from build123d import *

# Parameters (mm, degrees)
F0_W      = 184.15
F0_H      = 50.8
F1_DEPTH  = 8.128
F3_D      = 5.1054
F6_D      = 4.9784
F7_W      = 76.2
F7_H      = 9.525
F8_DEPTH  = 8.129
F9_SIZE   = 9.525
F10_SIZE  = 2.54
F15_DEPTH = 25.4
F17_D     = 5.1054
F18_R     = 2.4892
F19_DEPTH = 4.064
F20_SIZE  = 4.06399


# Not quite as in the source:
# - a fillet or chamfer is up to 0.001 mm smaller than in the source, because OpenCascade refuses the exact size
# - a feature names something its author has since deleted; it is built from what else it names


with BuildPart() as f1:
    # F0 (on Top) → F1 (new body)
    with BuildSketch(Plane.XY):
        Rectangle(F0_W, F0_H)
    extrude(amount=F1_DEPTH)

    # F3 (through all)
    with Locations(Plane.XY.offset(8.128)):
        with Locations((-60.325, 12.7), (-76.2, -12.7), (-44.45, -12.7)):
            Hole(F3_D / 2)

    # F6 (through all)
    with Locations(Plane.XY.offset(8.128)):
        with Locations((79.375, 12.7), (79.375, -12.7)):
            Hole(F6_D / 2)

    # F7 (on face) → F8 (cut, through all)
    with BuildSketch(Plane.XY.offset(8.128)):
        Polygon((66.675, 25.4), (-47.625, 25.4), (-34.925, 12.7), (53.975, 12.7), align=None)
        with Locations((15.875, -4.7625)):
            Rectangle(F7_W, F7_H)
    extrude(amount=-F8_DEPTH, mode=Mode.SUBTRACT)

    # F9
    f9_edges = [f1.edges().sort_by_distance(p)[0] for p in [
        (-92.075, -25.4, 4.064),
        (-92.075, 25.4, 4.064),
        (92.075, -25.4, 4.064),
        (92.075, 25.4, 4.064),
    ]]
    chamfer(f9_edges, length=F9_SIZE)

    # F10
    f10_edges = [f1.edges().sort_by_distance(p)[0] for p in [
        (-22.225, 0, 4.064),
        (-22.225, -9.525, 4.064),
        (53.975, 0, 4.064),
        (53.975, -9.525, 4.064),
    ]]
    chamfer(f10_edges, length=F10_SIZE)


with BuildPart() as f13_1:
    # F13: instance of F1
    add(f1.part.mirror(Plane(origin=(92.075, 0, 4.064), x_dir=(0, 1, 0), z_dir=(1, 0, 0))))

    # F17 (through all)
    with Locations(Plane.XY.offset(8.128)):
        with Locations((244.475, -6.35)):
            Hole(F17_D / 2)

    # F18 (on face) → F19 (cut)
    with BuildSketch(Plane(origin=(0, 0, 0), x_dir=(1, 0, 0), z_dir=(0, 0, -1))):
        Polygon((125.095, 25.4), (117.475, 25.4), (101.6, 25.4), (92.075, 15.875), (92.075, -15.875), (101.6, -25.4), (117.475, -25.4), (125.095, -17.78), align=None)
        with Locations((104.775, -12.7)):
            Circle(F18_R, mode=Mode.SUBTRACT)
        with Locations((104.775, 12.7)):
            Circle(F18_R, mode=Mode.SUBTRACT)
    extrude(amount=-F19_DEPTH, mode=Mode.SUBTRACT)

    # F20 (size 4.064 in the source; OpenCascade refuses exactly that, so slightly less here)
    f20_edges = [f13_1.edges().sort_by_distance(p)[0] for p in [
        (125.095, -3.81, 4.064),
    ]]
    chamfer(f20_edges, length=F20_SIZE)


with BuildPart() as f1_1:
    add(f1.part)

    # F14 (on face) → F15 (cut)
    with BuildSketch(Plane.XY.offset(8.128)):
        Polygon((-100.5587801337, -25.4), (92.075, -25.4), (92.075, -15.875), (92.075, 15.875), (92.075, 34.0131297708), (-100.5587801337, 34.0131297708), align=None)
    extrude(amount=-F15_DEPTH, mode=Mode.SUBTRACT)


solid = f13_1.part
Input: part model. Units: mm. Frame: model coordinates. A direction names the side the tool comes from. Give positions to 0.01 mm unless a question says otherwise; leave off trailing zeros. Loops run counter-clockwise (first coordinate to the right, second up) from the corner with the lowest first, then second, coordinate; pieces in that order, holes last. Notation, with made-up numbers: M -9.75,-32 L 5.25,-32 A12 ccw 5.25,-22 Z; hole C 30.25,66 d9. An arc over 180 degrees is marked long. Use CSV: the item, a comma, the result in double quotes.
(1) Section A-A, the plane y = -12.7. Count the separate pieces of the cut face and the enclosed holes in it, plus the area to 3 significant figures.
Outcome:
separate pieces,"4"
enclosed holes,"0"
area,"1,270 mm²"
(2) Section C-C, the plane x = 260.35. Return loops of the section in (y, z).
Outcome:
outline,"M -25.4,0 L -15.25,0 L -15.25,8.13 L -25.4,8.13 Z; M -10.15,0 L 25.4,0 L 25.4,8.13 L -10.15,8.13 Z"
(3) Pull-direction query (X, two-part tool) for faces 4 (the face through (130.175, -5, 4)), 5 (the face through (169, -9.525, 4)), 6 (the face through (185.4, 0.4, 8.128)), 7 (the face through (123.035, -1.447, 2.06)); classes: pulls with the +X half, pulls with the -X half, needs draft (parallel to the pull), parting line crosses it, or undercut.
Outcome:
face 4,"undercut"
face 5,"undercut"
face 6,"needs draft"
face 7,"pulls with the -X half"
(4) Set-up query: faces 1 (the face through (169, 0, 4)), 2 (the face through (125.325, 17.55, 5.024)), 3 (the face through (185, -25.4, 4)). Return all of +Z, -Z, +X, -X, +Y, -Y with unobstructed straight access to the full face (end or side cutting, diameter ignored); none if empty.
Outcome:
face 1,"+Z, -Z"
face 2,"+Z, -Z, +Y"
face 3,"+Z, -Z, +X, -X, -Y"
(5) Pin query (flat end, axial travel): P1, Ø8.5, axis at x = 110.5, y = 1, coming from the -Z side; P2, Ø2.5, axis at x = 168, z = 5.5, coming from the +Y side. Return the tip coordinate at first contact, or that it passes through.
Outcome:
P1,"stops at z = 4.06"
P2,"stops at y = 12.7"
(6) Section B-B, the plane x = 151.5. Return loops of the section in (y, z) (3 decimals), plus the area to 3 significant figures.
Outcome:
outline,"M -25.4,0 L -9.525,0 L -9.525,8.128 L -25.4,8.128 Z; M 0,0 L 12.7,0 L 12.7,8.128 L 0,8.128 Z"
area,"232 mm²"
(7) Material intervals for L1, parallel to Y at x = 149, z = 4.5 (3 decimals); L2, parallel to Y at x = 103, z = 4.5; L3, parallel to X at y = -15, z = 0.75 (3 decimals), sorted ascending. Write a range as [from, to].
Outcome:
L1,"y = [-25.4, -9.525], [0, 12.7]"
L2,"y = [-25.4, -14.45], [-10.95, 10.95], [14.45, 25.4]"
L3,"x = [124.345, 227.493], [229.707, 259.243], [261.457, 276.225]"
